The model under review builds one solid part; all positions refer to its coordinate system, in mm. A direction names the side the tool comes from. Round coordinates to 2 decimals unless told otherwise and drop trailing zeros. Order: outer loops, then holes, each group sorted by start corner. A loop starts at its lowest first (then second) coordinate and runs counter-clockwise, first axis right, second up.
```python
from build123d import *

# Parameters (mm, degrees)
SKETCH2_R           = 2
BOSS_EXTRUDE1_DEPTH = 20
SKETCH3_R           = 2
CUT_EXTRUDE1_DEPTH  = 10


with BuildPart() as part:
    # Sketch2 → Boss-Extrude1 (new, symmetric)
    with BuildSketch(Plane(origin=(0, 0, 0), x_dir=(0, 0, -1), z_dir=(1, 0, 0))):
        with BuildLine():
            Line((-1.5, 21.918644487), (-1.5, -8.081355513))
            Line((-1.5, -8.081355513), (1.5, -8.081355513))
            Line((1.5, -8.081355513), (1.5, 21.918644487))
            ThreePointArc((1.5, 21.918644487), (0, 31.688340494), (-1.5, 21.918644487))
        make_face()
        with Locations((0, 26.688340494)):
            Circle(SKETCH2_R, mode=Mode.SUBTRACT)
    extrude(amount=BOSS_EXTRUDE1_DEPTH, both=True)

    # Sketch3 → Cut-Extrude1 (cut, symmetric)
    with BuildSketch(Plane(origin=(0, 0, 0), x_dir=(0, 0, -1), z_dir=(1, 0, 0))):
        with BuildLine():
            Line((1.5, 21.918644487), (-1.5, 21.918644487))
            ThreePointArc((-1.5, 21.918644487), (0, 31.688340494), (1.5, 21.918644487))
        make_face()
        with Locations((0, 26.688340494)):
            Circle(SKETCH3_R, mode=Mode.SUBTRACT)
    extrude(amount=CUT_EXTRUDE1_DEPTH, both=True, mode=Mode.SUBTRACT)


solid = part.part
```
(1) Consider section B-B (y = 23.5). Write out the cut boundary in (x, z).
Data:
outline: (-20, -3.85) - (-10, -3.85) - (-10, 3.85) - (-20, 3.85) - close; (10, -3.85) - (20, -3.85) - (20, 3.85) - (10, 3.85) - close
(2) Draft analysis for pull direction Y (two halves, no side actions). For faces 4 (the cylindrical face through (-15.07, 28.67, 0.26)), 5 (the cylindrical face through (-14.93, 31.684, -0.199)), 6 (the flat face through (0, 21.919, 0)), 7 (the flat face through (-20, 17, 0)), state which applies: pulls with the +Y half, pulls with the -Y half, needs draft (parallel to the pull), parting line crosses it, or undercut.
Data:
face 4: undercut
face 5: parting line crosses it
face 6: pulls with the +Y half
face 7: needs draft
(3) Consider section D-D (y = 7). Write out the cut boundary in (x, z), and give its area (3 significant figures).
Data:
outline: (-20, -1.5) - (20, -1.5) - (20, 1.5) - (-20, 1.5) - close
area: 120 mm2
(4) For faces 1 (the flat face through (10, 26.9, 2.2)), 2 (the flat face through (0, 7, 1.5)), 3 (the flat face through (0, 7, -1.5)), list the 3-axis set-ups (+Z, -Z, +X, -X, +Y, -Y) from which the entire face can be reached by the end or side of a thin tool; tool diameter is ignored.
Data:
face 1: +Z, -Z, +Y
face 2: +Z, +X, -X, -Y
face 3: -Z, +X, -X, -Y
(5) Consider section C-C (z = -4). Write out the cut boundary in (x, y), and give its area (3 significant figures).
Data:
outline: (-20, 23.69) - (-10, 23.69) - (-10, 29.69) - (-20, 29.69) - close; (10, 23.69) - (20, 23.69) - (20, 29.69) - (10, 29.69) - close
area: 120 mm2
(6) To check wall thickness, follow probe 1 along X at (y, z) = (29.5, -0.5); probe 2 along Y at (x, z) = (-15.5, 0); probe 3 along Z at (x, y) = (0.5, 14). State the ranges of each line that lie inside material, in increasing order.
Data:
probe 1: x = -20 to -10, 10 to 20
probe 2: y = -8.08 to 24.69, 28.69 to 31.69
probe 3: z = -1.5 to 1.5
(7) Consider section A-A (z = 0). Write out the cut boundary in (x, y), and give its area (3 significant figures).
Data:
outline: (-20, -8.08) - (20, -8.08) - (20, 24.69) - (10, 24.69) - (10, 21.92) - (-10, 21.92) - (-10, 24.69) - (-20, 24.69) - close; (-20, 28.69) - (-10, 28.69) - (-10, 31.69) - (-20, 31.69) - close; (10, 28.69) - (20, 28.69) - (20, 31.69) - (10, 31.69) - close
area: 1,320 mm2
(8) Insertion check: pin 1 (15 mm diameter, centred on x = 9.5, y = 9, fed in from -Z); pin 2 (3 mm diameter, centred on x = 13.5, z = -3, fed in from +Y); pin 3 (2 mm diameter, centred on x = -16, z = 4, fed in from -Y); pin 4 (1 mm diameter, centred on y = 3.5, z = -3, fed in from +X). Each pin has a flat end and moves straight along its axis. Give the tip position at first contact, or say it passes through.
Data:
pin 1: stops at z = -1.5
pin 2: stops at y = 31.46
pin 3: stops at y = 22.69
pin 4: passes through
